```python
from build123d import *

# Parameters (mm, degrees)
SKETCH037_W     = 40
SKETCH037_H     = 40
SKETCH040_W     = 33
SKETCH040_H     = 33
POCKET025_DEPTH = 5
SKETCH039_R     = 1.65
POCKET026_DEPTH = 5
POCKET027_DEPTH = 5
FILLET001_R     = 2.5
CHAMFER011_SIZE = 3


with BuildPart() as part:
    # Sketch037 → AdditiveLoft section 0
    with BuildSketch(Plane.XY):
        Rectangle(SKETCH037_W, SKETCH037_H)
    # Sketch040 → AdditiveLoft section 1
    with BuildSketch(Plane.XY.offset(5.5)):
        Rectangle(SKETCH040_W, SKETCH040_H)
    loft()

    # Sketch038 → Pocket025 (cut)
    with BuildSketch(Plane.XY):
        with BuildLine():
            ThreePointArc((-12, 15.2), (-14.262742, 14.262742), (-15.2, 12))
            Line((-15.2, -12), (-15.2, 12))
            ThreePointArc((-15.2, -12), (-14.262742, -14.262742), (-12, -15.2))
            Line((12, -15.2), (-12, -15.2))
            ThreePointArc((12, -15.2), (14.262742, -14.262742), (15.2, -12))
            Line((15.2, 12), (15.2, -12))
            ThreePointArc((15.2, 12), (14.262742, 14.262742), (12, 15.2))
            Line((-12, 15.2), (12, 15.2))
        make_face()
    extrude(amount=POCKET025_DEPTH, mode=Mode.SUBTRACT)

    # Sketch039 → Pocket026 (cut)
    with BuildSketch(Plane.XY.offset(5.5)):
        with Locations((-12, 12)):
            Circle(SKETCH039_R)
        with Locations((12, 12)):
            Circle(SKETCH039_R)
        with Locations((12, -12)):
            Circle(SKETCH039_R)
        with Locations((-12, -12)):
            Circle(SKETCH039_R)
    extrude(amount=-POCKET026_DEPTH, mode=Mode.SUBTRACT)

    # Sketch041 → Pocket027 (cut)
    with BuildSketch(Plane.XY.offset(5.5)):
        with BuildLine():
            ThreePointArc((10.891901, 9.265878), (0, 14.3), (-10.891901, 9.265878))
            ThreePointArc((-10.891901, 9.265878), (-11.123261, 8.500069), (-10.71909, 7.80968))
            Line((-10.71909, 7.80968), (-7.63557, 5.563099))
            ThreePointArc((-7.63557, 5.563099), (-6.943871, 5.376635), (-6.30495, 5.700667))
            ThreePointArc((6.30495, 5.700667), (0, 8.5), (-6.30495, 5.700667))
            ThreePointArc((6.30495, 5.700667), (6.943871, 5.376635), (7.63557, 5.563099))
            Line((10.71909, 7.80968), (7.63557, 5.563099))
            ThreePointArc((10.71909, 7.80968), (11.123261, 8.500069), (10.891901, 9.265878))
        make_face()
        with BuildLine():
            ThreePointArc((-13.470436, 4.799724), (-12.384163, -7.15), (-2.578535, -14.065602))
            ThreePointArc((-2.578535, -14.065602), (-1.799645, -13.883061), (-1.403836, -13.187845))
            Line((-1.403836, -13.187845), (-1, -9.394147))
            ThreePointArc((-1, -9.394147), (-1.184367, -8.701886), (-1.784447, -8.310581))
            ThreePointArc((-8.089397, 2.609914), (-7.361216, -4.25), (-1.784447, -8.310581))
            ThreePointArc((-8.089397, 2.609914), (-8.128238, 3.325251), (-8.63557, 3.831048))
            Line((-12.122927, 5.378164), (-8.63557, 3.831048))
            ThreePointArc((-12.122927, 5.378164), (-12.922906, 5.382992), (-13.470436, 4.799724))
        make_face()
        with BuildLine():
            ThreePointArc((2.578535, -14.065602), (12.384163, -7.15), (13.470436, 4.799724))
            ThreePointArc((13.470436, 4.799724), (12.922906, 5.382992), (12.122927, 5.378164))
            Line((8.63557, 3.831048), (12.122927, 5.378164))
            ThreePointArc((8.63557, 3.831048), (8.128238, 3.325251), (8.089397, 2.609914))
            ThreePointArc((1.784447, -8.310581), (7.361216, -4.25), (8.089397, 2.609914))
            ThreePointArc((1.784447, -8.310581), (1.184367, -8.701886), (1, -9.394147))
            Line((1, -9.394147), (1.403836, -13.187845))
            ThreePointArc((1.403836, -13.187845), (1.799645, -13.883061), (2.578535, -14.065602))
        make_face()
    extrude(amount=-POCKET027_DEPTH, mode=Mode.SUBTRACT)

    # Fillet001
    fillet001_edges = [part.edges().sort_by_distance(p)[0] for p in [
        (18.25, -18.25, 2.75),
        (18.25, 18.25, 2.75),
        (-18.25, -18.25, 2.75),
        (-18.25, 18.25, 2.75),
        (16.5, 0, 5.5),
        (0, -16.5, 5.5),
        (-16.5, 0, 5.5),
        (0, 16.5, 5.5),
    ]]
    fillet(fillet001_edges, radius=FILLET001_R)

    # Chamfer011
    chamfer011_edges = [part.edges().sort_by_distance(p)[0] for p in [
        (14.262742, 14.262742, 0),
    ]]
    chamfer(chamfer011_edges, length=CHAMFER011_SIZE)


with BuildPart() as part_1:
    # Body002 placement: moved
    add(part.part.moved(Location((6, 2, 25.3))))


solid = part_1.part
```
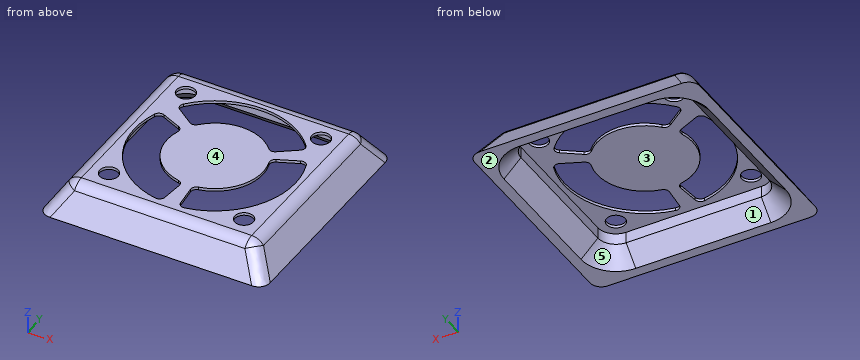
Can you work these out from the model? Positions are in its coordinate system, mm. Face numbers are marked on the shaded views. A direction names the side the tool comes from. Give positions to 0.01 mm unless a question says otherwise; leave off trailing zeros. One line per question, with ' | ' between items. Start each with the question number.
Q1. If I drill on line 1 (Y direction, x = -6, z = 30.5); line 2 (Z direction, x = 20, y = -12); line 3 (Y direction, x = -6, z = 30.6), over which ranges is the centre line in solid material (lowest first)? Write a range as from..to.
Q2. For the marked faces 1 and 2, which set-ups out of +Z, -Z, +X, -X, +Y, -Y let a thin tool reach every point of the face, with its end or its side?
Q3. If we mould it in two halves opening along Y, with no side actions, what happens to the marked faces 3, 4 and 5? For each: +Y half, -Y half, draft (parallel to the pull), parting line (faces both ways), or undercut.
Q4. For pin 1 Ø1 at (x, y) = (13.5, -4) entering from +Z; pin 2 Ø4 at (x, y) = (18, -10) entering from -Z; pin 3 Ø1 at (y, z) = (2, 29.5) entering from +X; pin 4 Ø1 at (y, z) = (0.5, 29) entering from -X, each with a flat end and sliding along its axis, tell me the tip position at first contact or that it passes through.
Q5. If we section it at A-A (y = -3): State how many separate pieces and enclosed holes the cut face has, plus the area to 3 significant figures.
Computed:
1) line 1: y = -14.32..-11.65, -8.35..-5.78, 7.32..12.35, 15.65..18.32 | line 2: z = 30.3..30.8 | line 3: y = -14.11..-11.65, -8.35..-5.78, 7.32..12.35, 15.65..18.11
2) face 1: -Z | face 2: -Z, +X, -X, +Y, -Y
3) face 3: undercut | face 4: draft | face 5: undercut
4) pin 1: passes through | pin 2: stops at z = 30.3 | pin 3: stops at x = 23.65 | pin 4: stops at x = -11.96
5) separate pieces: 3 | enclosed holes: 0 | area: 32.6 mm²
